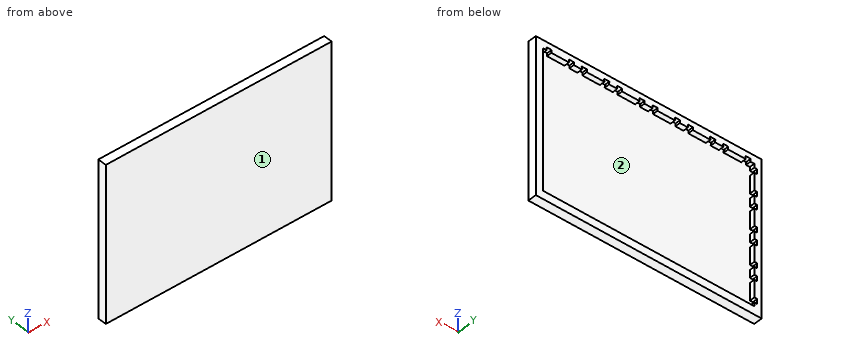
from build123d import *

# Parameters (mm, degrees)
SKETCH1_W           = 131
SKETCH1_H           = 91
BOSS_EXTRUDE1_DEPTH = 5
CUT_EXTRUDE2_DEPTH  = 3


with BuildPart() as part:
    # Sketch1 → Boss-Extrude1 (new body)
    with BuildSketch(Plane(origin=(0, 0, 0), x_dir=(1, 0, 0), z_dir=(0, 1, 0))):
        Rectangle(SKETCH1_W, SKETCH1_H)
    extrude(amount=BOSS_EXTRUDE1_DEPTH)

    # Sketch3 → Cut-Extrude2 (cut)
    with BuildSketch(Plane(origin=(0, 5, 0), x_dir=(1, 0, 0), z_dir=(0, 1, 0))):
        Polygon((-61.25, -40.75), (-59.05, -40.75), (-59.15, -42.45), (-56.15, -42.45), (-56.25, -40.75), (-46.05, -40.75), (-46.15, -42.45), (-43.15, -42.45), (-43.25, -40.75), (-38.55, -40.75), (-38.65, -42.45), (-35.65, -42.45), (-35.75, -40.75), (-25.55, -40.75), (-25.65, -42.45), (-22.65, -42.45), (-22.75, -40.75), (-18.05, -40.75), (-18.15, -42.45), (-15.15, -42.45), (-15.25, -40.75), (-5.05, -40.75), (-5.15, -42.45), (-2.15, -42.45), (-2.25, -40.75), (2.45, -40.75), (2.35, -42.45), (5.35, -42.45), (5.25, -40.75), (15.45, -40.75), (15.35, -42.45), (18.35, -42.45), (18.25, -40.75), (22.95, -40.75), (22.85, -42.45), (25.85, -42.45), (25.75, -40.75), (35.95, -40.75), (35.85, -42.45), (38.85, -42.45), (38.75, -40.75), (43.45, -40.75), (43.35, -42.45), (46.35, -42.45), (46.25, -40.75), (56.45, -40.75), (56.35, -42.45), (59.35, -42.45), (59.25, -40.75), (61.25, -40.75), (61.25, 40.75), (-61.25, 40.75), (-61.25, 38.55), (-62.95, 38.65), (-62.95, 35.65), (-61.25, 35.75), (-61.25, 25.55), (-62.95, 25.65), (-62.95, 22.65), (-61.25, 22.75), (-61.25, 18.116666667), (-62.95, 18.216666667), (-62.95, 15.216666667), (-61.25, 15.316666667), (-61.25, 5.116666667), (-62.95, 5.216666667), (-62.95, 2.216666667), (-61.25, 2.316666667), (-61.25, -2.316666667), (-62.95, -2.216666667), (-62.95, -5.216666667), (-61.25, -5.116666667), (-61.25, -15.316666667), (-62.95, -15.216666667), (-62.95, -18.216666667), (-61.25, -18.116666667), (-61.25, -22.75), (-62.95, -22.65), (-62.95, -25.65), (-61.25, -25.55), (-61.25, -35.75), (-62.95, -35.65), (-62.95, -38.65), (-61.25, -38.55), align=None)
    extrude(amount=-CUT_EXTRUDE2_DEPTH, mode=Mode.SUBTRACT)


solid = part.part
Can you work these out from the model? Positions are in its coordinate system, mm. Face numbers are marked on the shaded views. Round coordinates to 2 decimals unless told otherwise and drop trailing zeros. Order: outer loops, then holes, each group sorted by start corner. A loop starts at its lowest first (then second) coordinate and runs counter-clockwise, first axis right, second up. Notation, with made-up numbers: (17.25, 40) - (62.25, 40) arc R20 ccw to (62.25, 62) - close; hole circle Ø11 at (-13.5, 70.5). An arc over 180 degrees is marked (long way). Answer in a Markdown table with one row per item.
(1) For P1, Ø10, axis at x = 51, z = -5, coming from the +Y side, with a flat end and sliding along its axis, tell me the tip position at first contact or that it passes through.
From the geometry:
| item | result |
|---|---|
| P1 | stops at y = 2 |
(2) Please list where these lines run through material, in increasing order: L1, parallel to Z at x = 27.5, y = 4.85; L2, parallel to X at y = 3.5, z = -22; L3, parallel to Z at x = -18, y = 2.15. Write a range as from..to.
From the geometry:
| item | result |
|---|---|
| L1 | z = -45.5..-40.75, 40.75..45.5 |
| L2 | x = -65.5..-61.25, 61.25..65.5 |
| L3 | z = -45.5..-40.75, 42.45..45.5 |
(3) If we mould it in two halves opening along X, with no side actions, what happens to the marked faces 1 and 2? For each: released by +X, released by -X, zero draft, split by the parting line, or undercut.
From the geometry:
| item | result |
|---|---|
| face 1 | zero draft |
| face 2 | undercut |
(4) Suppose I cut it at A-A, the plane x = 21.5. Please give me the cut outline in (y, z), plus the area to 4 significant figures.
From the geometry:
| item | result |
|---|---|
| outline | (0, -45.5) - (5, -45.5) - (5, -40.75) - (2, -40.75) - (2, 40.75) - (5, 40.75) - (5, 45.5) - (0, 45.5) - close |
| area | 210.5 mm2 |
(5) Suppose I cut it at B-B, the plane z = -8. Please give me the cut outline in (x, y).
From the geometry:
| item | result |
|---|---|
| outline | (-65.5, 0) - (65.5, 0) - (65.5, 5) - (61.25, 5) - (61.25, 2) - (-61.25, 2) - (-61.25, 5) - (-65.5, 5) - close |
